Can you work these out from the model? Positions are in its coordinate system, mm. Face numbers are marked on the shaded views. A direction names the side the tool comes from. Round coordinates to 2 decimals unless told otherwise and drop trailing zeros. Write each loop counter-clockwise with the first axis right and the second up, starting at its lowest first coordinate (ties: lowest second). Pieces come first, ordered by that corner, then holes.
Q1. If we section it at A-A (y = 0): Please give me the cut outline in (x, z) (3 decimals).
Q2. Please list where these lines run through material, in increasing order: line 1 along Y through (x, z) = (-4.25, 0) (3 decimals); line 2 along Y through (x, z) = (-19, 0); line 3 along X through (y, z) = (-5.5, 4).
Q3. For the marked faces 4 and 5, which set-ups out of +Z, -Z, +X, -X, +Y, -Y let a thin tool reach every point of the face, with its end or its side?
Q4. If we section it at C-C (x = -18): Please give me the cut outline in (y, z).
Q5. I'm going to push flat-ended pins straight in: pin 1 Ø4 at (x, y) = (-15.5, -5) entering from +Z; pin 2 Ø1 at (x, y) = (-6, -2) entering from -Z; pin 3 Ø5 at (x, y) = (-2.5, -8) entering from -Z; pin 4 Ø6 at (x, z) = (-18.5, 7) entering from -Y (3 decimals). Where does each tip first touch, or does it pass through?
Q6. We'd pull the mould along Y, two halves only. Please class the marked faces 1, 2 and 3: +Y half, -Y half, draft (parallel to the pull), parting line (faces both ways), or undercut.
Q7. If we section it at D-D (x = -14): Please give me the cut outline in (y, z), plus the area to 3 significant figures.
from build123d import *


with BuildPart() as part:
    # Sketch1 → Revolve1 (revolve)
    with BuildSketch(Plane(origin=(0, 0, 0), x_dir=(1, 0, 0), z_dir=(0, 1, 0))):
        with BuildLine():
            Line((-14.8, 11.65), (-14.8, 3.15))
            ThreePointArc((-14.8, 3.15), (-15.239339828, 2.089339828), (-16.3, 1.65))
            Line((-16.3, 1.65), (-20.8, 1.65))
            Line((-20.8, 1.65), (-21.8, 1.09375))
            Line((-21.8, 1.09375), (-21.8, 0.79375))
            Line((-21.8, 0.79375), (-9.8, 0.79375))
            Line((-9.8, 0.79375), (-9.8, 4.225))
            Line((-9.8, 4.225), (0, 4.225))
            Line((0, 4.225), (0, 10))
            Line((0, 10), (-10.3, 10))
            ThreePointArc((-10.3, 10), (-11.360660172, 10.439339828), (-11.8, 11.5))
            Line((-11.8, 11.5), (-11.8, 11.65))
            Line((-11.8, 11.65), (-14.8, 11.65))
        make_face()
    revolve(axis=Axis((-74.867571618, 0, 0), (1, 0, 0)))


solid = part.part
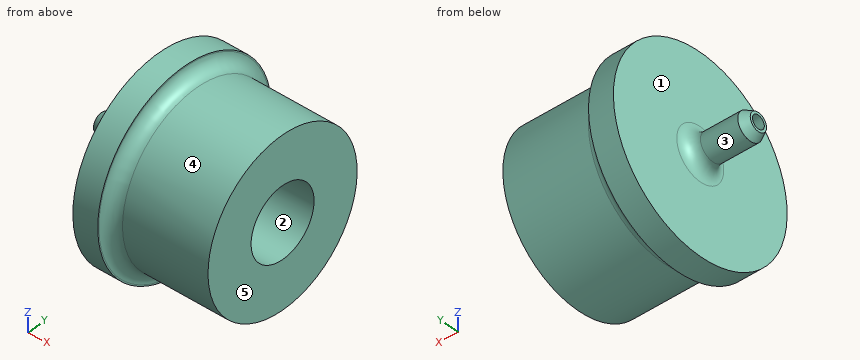
A:
1. outline: (-21.8, -1.094) - (-20.8, -1.65) - (-16.3, -1.65) arc R1.5 cw to (-14.8, -3.15) - (-14.8, -11.65) - (-11.8, -11.65) - (-11.8, -11.5) arc R1.5 cw to (-10.3, -10) - (0, -10) - (0, -4.225) - (-9.8, -4.225) - (-9.8, -0.794) - (-21.8, -0.794) - close; (-21.8, 0.794) - (-9.8, 0.794) - (-9.8, 4.225) - (0, 4.225) - (0, 10) - (-10.3, 10) arc R1.5 cw to (-11.8, 11.5) - (-11.8, 11.65) - (-14.8, 11.65) - (-14.8, 3.15) arc R1.5 cw to (-16.3, 1.65) - (-20.8, 1.65) - (-21.8, 1.094) - close
2. line 1: y = -10 to -4.225, 4.225 to 10
2. line 2: y = -1.65 to -0.79, 0.79 to 1.65
2. line 3: x = -14.8 to 0
3. face 4: +X
3. face 5: +Z, -Z, +X, +Y, -Y
4. outline: circle Ø3.3 at (0, 0); hole circle Ø1.59 at (0, 0)
5. pin 1: stops at z = 11.22
5. pin 2: stops at z = -9.89
5. pin 3: stops at z = -8.35
5. pin 4: passes through
6. face 1: draft
6. face 2: undercut
6. face 3: parting line
7. outline: circle Ø23.3 at (0, 0); hole circle Ø1.59 at (0, 0)
7. area: 424 mm2
